Could you check a few things on this drawing? It's one solid part, dimensions in mm from its lowest x, y, z. Round coordinates to 2 decimals unless told otherwise and drop trailing zeros. Write each loop counter-clockwise with the first axis right and the second up, starting at its lowest first coordinate (ties: lowest second). Pieces come first, ordered by that corner, then holes. Notation, with made-up numbers: (41.5, -16.5) -> (71.5, -16.5) arc R11 ccw to (71.5, 4.5) -> close; hole circle Ø5 at (69, 36). An arc over 180 degrees is marked (long way). Return JSON: item names as keys, results as strings.
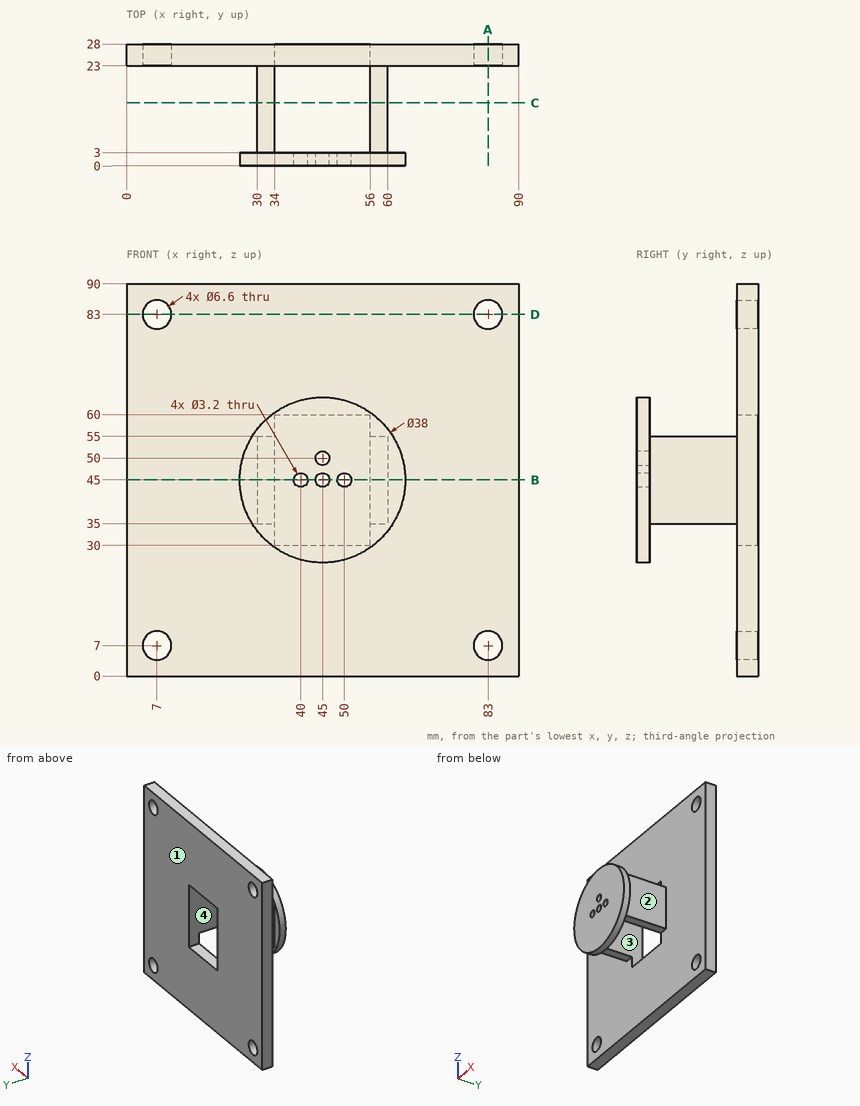
1) I want a section at C-C, the plane y = 14.5. Please give me the cut outline in (x, z), and give its area (3 significant figures).
Return value:
{"outline": "(30, 35) -> (34, 35) -> (34, 55) -> (30, 55) -> close; (56, 35) -> (60, 35) -> (60, 55) -> (56, 55) -> close", "area": "160 mm²"}
2) I want a section at A-A, the plane x = 83. Please give me the cut outline in (y, z), and give its area (3 significant figures).
Return value:
{"outline": "(23, 0) -> (28, 0) -> (28, 3.7) -> (23, 3.7) -> close; (23, 10.3) -> (28, 10.3) -> (28, 79.7) -> (23, 79.7) -> close; (23, 86.3) -> (28, 86.3) -> (28, 90) -> (23, 90) -> close", "area": "384 mm²"}
3) I want a section at B-B, the plane z = 45. Please give me the cut outline in (x, y), and give its area (3 significant figures).
Return value:
{"outline": "(0, 23) -> (30, 23) -> (30, 3) -> (26, 3) -> (26, 0) -> (38.4, 0) -> (38.4, 3) -> (34, 3) -> (34, 28) -> (0, 28) -> close; (41.6, 0) -> (43.4, 0) -> (43.4, 3) -> (41.6, 3) -> close; (46.6, 0) -> (48.4, 0) -> (48.4, 3) -> (46.6, 3) -> close; (51.6, 0) -> (64, 0) -> (64, 3) -> (60, 3) -> (60, 23) -> (90, 23) -> (90, 28) -> (56, 28) -> (56, 3) -> (51.6, 3) -> close", "area": "585 mm²"}
4) Thinking about a two-plate mould opening in X: for the marked faces 1, 2, 3 and 4, which applies, pulls with the +X half, pulls with the -X half, needs draft (parallel to the pull), parting line crosses it, or undercut?
Return value:
{"face 1": "needs draft", "face 2": "pulls with the +X half", "face 3": "undercut", "face 4": "undercut"}
5) Will these pins go through, and if not, where does the flat tip stop? pin 1 Ø2 at (x, y) = (31, 10) entering from -Z; pin 2 Ø10 at (x, y) = (59.5, 10) entering from +Z; pin 3 Ø5 at (x, z) = (12, 80) entering from -Y.
Return value:
{"pin 1": "z = 35", "pin 2": "z = 55", "pin 3": "y = 23"}
6) If I drill on probe 1 along Z at (x, y) = (7, 26.75); probe 2 along X at (y, z) = (3.5, 54.5), over which ranges is the centre line in solid material (lowest first)? Write a range as [from, to].
Return value:
{"probe 1": "[0, 3.7], [10.3, 79.7], [86.3, 90]", "probe 2": "[30, 34], [56, 60]"}
7) I want a section at D-D, the plane z = 83. Please give me the cut outline in (x, y), and give its area (3 significant figures).
Return value:
{"outline": "(0, 23) -> (3.7, 23) -> (3.7, 28) -> (0, 28) -> close; (10.3, 23) -> (79.7, 23) -> (79.7, 28) -> (10.3, 28) -> close; (86.3, 23) -> (90, 23) -> (90, 28) -> (86.3, 28) -> close", "area": "384 mm²"}
